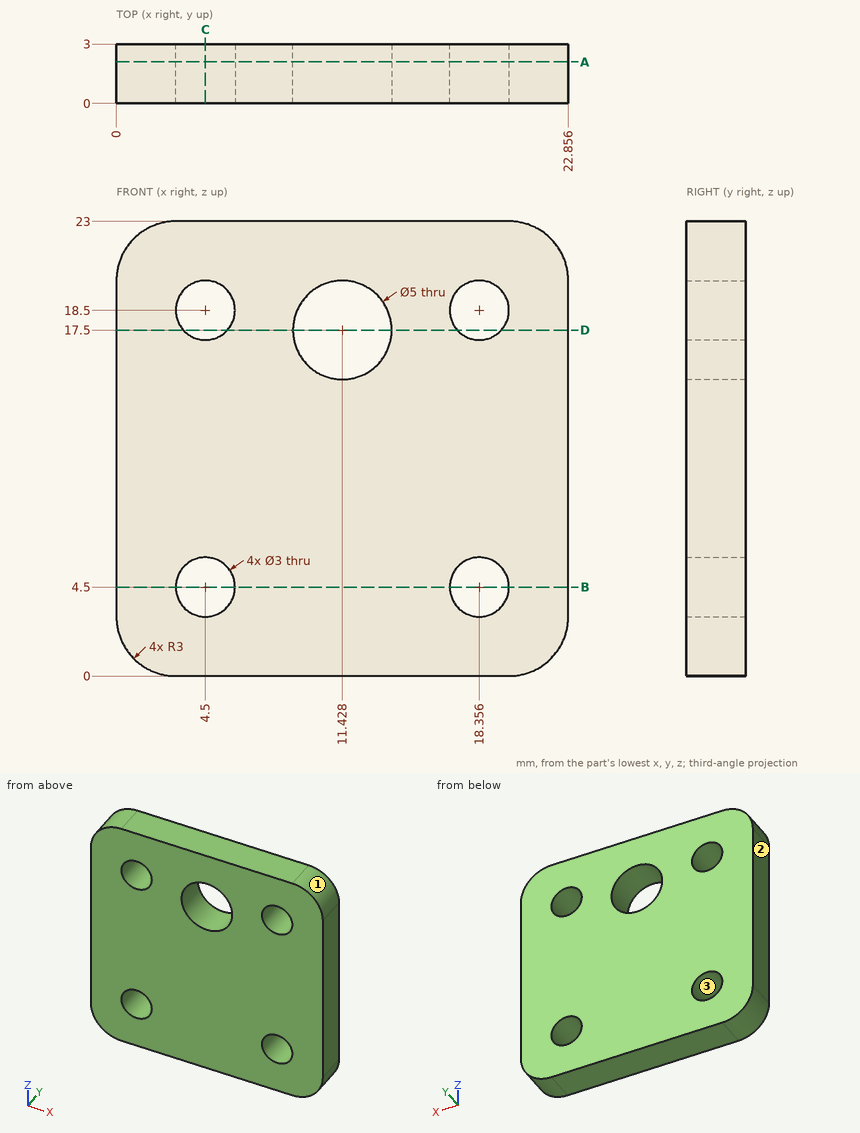
Verification items for this drawing (mm, ordinates from the low corner). Round coordinates to 2 decimals unless told otherwise and drop trailing zeros. Loops run counter-clockwise (first coordinate to the right, second up) from the corner with the lowest first, then second, coordinate; pieces in that order, holes last. Notation, with made-up numbers: (-35, 41.25) -> (11, 41.25) arc R12 cw to (11, 60.25) -> close; hole circle Ø9 at (0.5, -33.5). An arc over 180 degrees is marked (long way). Write item = value, one per line. Start each with the question number.
1) Gauge pin test, flat ends, axial feed: pin 1 Ø3.5 at (x, z) = (4.5, 4.5) entering from +Y; pin 2 Ø4 at (x, z) = (11.43, 17.5) entering from -Y. Record the tip position at first contact, or that the pin passes through.
2) Release check for a two-part mould opening along Z. For the marked faces 1, 2 and 3 record: released by +Z, released by -Z, zero draft, split by the parting line, or undercut.
3) Thickness scan on probe 1 along Z at (x, y) = (17, 0.8); probe 2 along Z at (x, y) = (19.25, 0.7) (1 decimal); probe 3 along X at (y, z) = (0.6, 4.75) (1 decimal). Record the ranges inside material, lowest first.
4) Sectioned sample at C-C, the plane x = 4.5. Record the cut outline in (y, z), plus the area to 3 significant figures.
5) Sectioned sample at D-D, the plane z = 17.5. Record the cut outline in (x, y) (1 decimal).
6) Sectioned sample at A-A, the plane y = 2.1. Record the cut outline in (x, z).
7) Sectioned sample at B-B, the plane z = 4.5. Record the cut outline in (x, y).
Results are:
q1.pin_1 = 3
q1.pin_2 = through
q2.face_1 = released by +Z
q2.face_2 = zero draft
q2.face_3 = undercut
q3.probe_1 = 0 to 3.86, 5.14 to 17.86, 19.14 to 23
q3.probe_2 = 0 to 3.3, 5.7 to 17.3, 19.7 to 23
q3.probe_3 = 0 to 3, 6 to 16.9, 19.8 to 22.9
q4.outline = (0, 0) -> (3, 0) -> (3, 3) -> (0, 3) -> close; (0, 6) -> (3, 6) -> (3, 17) -> (0, 17) -> close; (0, 20) -> (3, 20) -> (3, 23) -> (0, 23) -> close
q4.area = 51.0 mm^2
q5.outline = (0, 0) -> (3.4, 0) -> (3.4, 3) -> (0, 3) -> close; (5.6, 0) -> (8.9, 0) -> (8.9, 3) -> (5.6, 3) -> close; (13.9, 0) -> (17.2, 0) -> (17.2, 3) -> (13.9, 3) -> close; (19.5, 0) -> (22.9, 0) -> (22.9, 3) -> (19.5, 3) -> close
q6.outline = (0, 3) arc R3 ccw to (3, 0) -> (19.86, 0) arc R3 ccw to (22.86, 3) -> (22.86, 20) arc R3 ccw to (19.86, 23) -> (3, 23) arc R3 ccw to (0, 20) -> close; hole circle Ø3 at (4.5, 4.5); hole circle Ø3 at (4.5, 18.5); hole circle Ø5 at (11.43, 17.5); hole circle Ø3 at (18.36, 4.5); hole circle Ø3 at (18.36, 18.5)
q7.outline = (0, 0) -> (3, 0) -> (3, 3) -> (0, 3) -> close; (6, 0) -> (16.86, 0) -> (16.86, 3) -> (6, 3) -> close; (19.86, 0) -> (22.86, 0) -> (22.86, 3) -> (19.86, 3) -> close
